Design review of the part shown in the three views and the two pictorial views. Dimensions are in mm from the part's minimum x, y and z. Round coordinates to 2 decimals unless told otherwise and drop trailing zeros. Loops run counter-clockwise (first coordinate to the right, second up) from the corner with the lowest first, then second, coordinate; pieces in that order, holes last. Notation, with made-up numbers: M 85.25,-17 L 122.25,-17 A20 cw 122.25,-1 Z; hole C -25.75,88.25 d6. An arc over 180 degrees is marked long. Return JSON: item names as keys, results as strings. Group by question number.
Q1. Consider section A-A (y = 4). State the section outline as (x, z) points (3 decimals).
Q2. Consider section C-C (z = 39.32). State the section outline as (x, y) points, and give its area (3 significant figures).
Q3. Consider section D-D (z = 48.5). State the section outline as (x, y) points.
Q4. To check wall thickness, follow line 1 along Y through (x, z) = (1.8, 66.5); line 2 along Y through (x, z) = (1.05, 10.5); line 3 along Z through (x, y) = (0.3, 13). State the ranges of each line that lie inside material, in increasing order.
Q5. Clearance check with a flat-ended pin moving along its axis: pin 1 Ø0.9 at (x, y) = (2, 4) entering from -Z. State where the tip first meets the part, or that it passes through.
Q6. Consider section B-B (x = 0.7). State the section outline as (y, z) points (1 decimal), and give its area (3 significant figures).
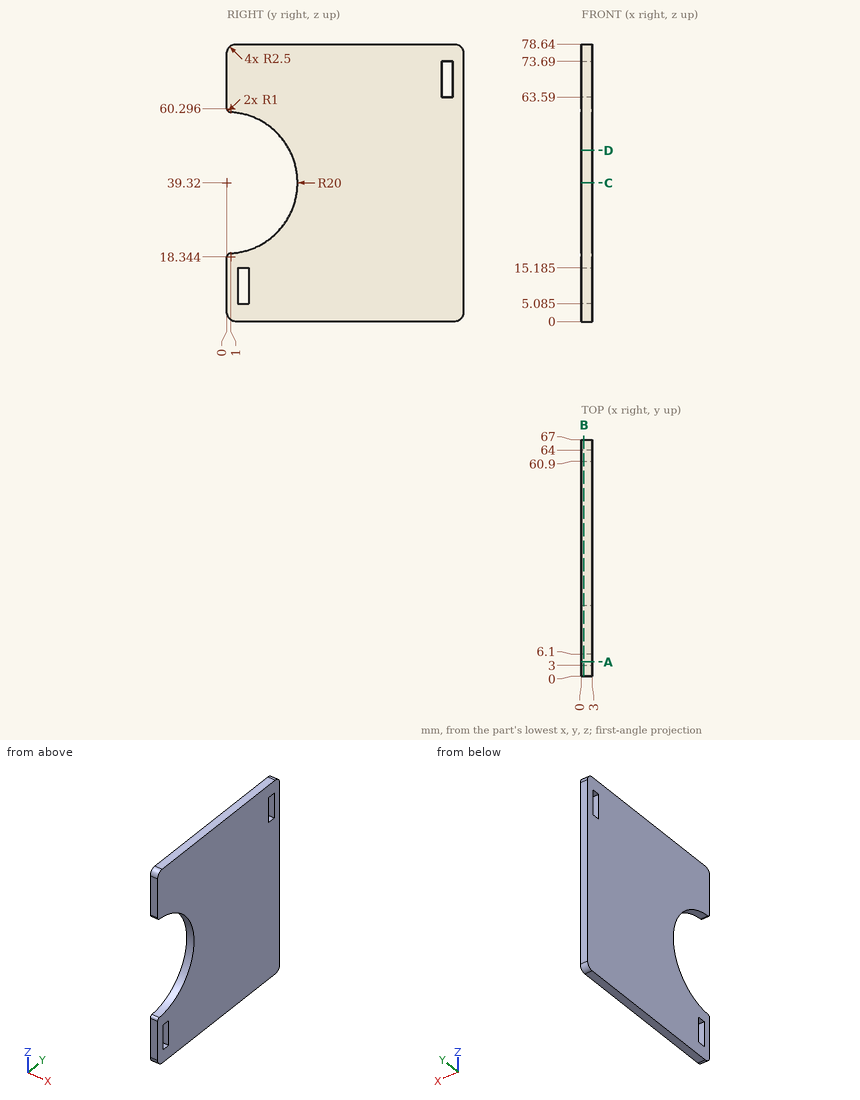
Values:
{
 "1": {"outline": "M 0,0 L 3,0 L 3,5.085 L 0,5.085 Z; M 0,15.185 L 3,15.185 L 3,19.724 L 0,19.724 Z; M 0,58.916 L 3,58.916 L 3,78.64 L 0,78.64 Z"},
 "2": {"outline": "M 0,20 L 3,20 L 3,67 L 0,67 Z", "area": "141 mm2"},
 "3": {"outline": "M 0,17.77 L 3,17.77 L 3,67 L 0,67 Z"},
 "4": {"line 1": "y = 0 to 60.9, 64 to 67", "line 2": "y = 0 to 3, 6.1 to 67", "line 3": "z = 0 to 24.12, 54.52 to 78.64"},
 "5": {"pin 1": "stops at z = 0"},
 "6": {"outline": "M 0,2.5 A2.5 ccw 2.5,0 L 64.5,0 A2.5 ccw 67,2.5 L 67,76.1 A2.5 ccw 64.5,78.6 L 2.5,78.6 A2.5 ccw 0,76.1 L 0,60.3 A1 ccw 1,59.3 A20 cw 1,19.3 A1 ccw 0,18.3 Z; hole M 3,5.1 L 6.1,5.1 L 6.1,15.2 L 3,15.2 Z; hole M 60.9,63.6 L 64,63.6 L 64,73.7 L 60.9,73.7 Z", "area": "4,570 mm2"}
}
